Could you check a few things on this model? Use its own coordinates, in mm. Face numbers are marked on the shaded views. A direction names the side the tool comes from. Give positions to 0.01 mm unless a question says otherwise; leave off trailing zeros. Loops run counter-clockwise (first coordinate to the right, second up) from the corner with the lowest first, then second, coordinate; pieces in that order, holes last. Notation, with made-up numbers: (-28, 41) -> (-20, 41) arc R16 ccw to (-20, 46) -> close; hole circle Ø4 at (40, 63). An arc over 180 degrees is marked (long way). Put each result on its own line as item: value.
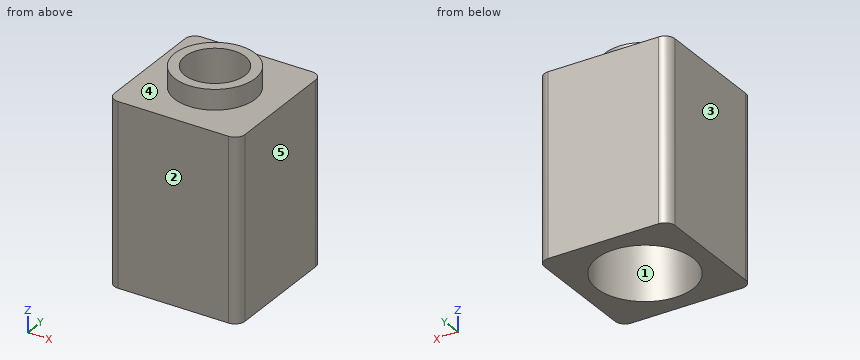
```python
from build123d import *

# Parameters (mm, degrees)
SKETCH2_R           = 1.5
BOSS_EXTRUDE1_DEPTH = 10
SKETCH3_R           = 2
CUT_EXTRUDE1_DEPTH  = 1
SKETCH4_R           = 2.4
CUT_EXTRUDE2_DEPTH  = 8


with BuildPart() as part:
    # Sketch2 → Boss-Extrude1 (new body)
    with BuildSketch(Plane(origin=(0, 0, -57.465471353), x_dir=(-1, 0, 0), z_dir=(0, 0, -1))):
        with BuildLine():
            Line((-6.490457264, -35.078386779), (-0.990457264, -35.078386779))
            ThreePointArc((-0.990457264, -35.078386779), (-0.636903873, -34.931940169), (-0.490457264, -34.578386779))
            Line((-0.490457264, -34.578386779), (-0.490457264, -29.078386779))
            ThreePointArc((-0.490457264, -29.078386779), (-0.636903873, -28.724833388), (-0.990457264, -28.578386779))
            Line((-0.990457264, -28.578386779), (-6.490457264, -28.578386779))
            ThreePointArc((-6.490457264, -28.578386779), (-6.844010654, -28.724833388), (-6.990457264, -29.078386779))
            Line((-6.990457264, -29.078386779), (-6.990457264, -34.578386779))
            ThreePointArc((-6.990457264, -34.578386779), (-6.844010654, -34.931940169), (-6.490457264, -35.078386779))
        make_face()
        with Locations((-3.740457264, -31.828386779)):
            Circle(SKETCH2_R, mode=Mode.SUBTRACT)
    extrude(amount=BOSS_EXTRUDE1_DEPTH)

    # Sketch3 → Cut-Extrude1 (cut)
    with BuildSketch(Plane(origin=(0, 0, -57.465471353), x_dir=(-1, 0, 0), z_dir=(0, 0, -1))):
        with BuildLine():
            Line((-0.990457264, -28.578386779), (-6.490457264, -28.578386779))
            ThreePointArc((-6.490457264, -28.578386779), (-6.844010654, -28.724833388), (-6.990457264, -29.078386779))
            Line((-6.990457264, -29.078386779), (-6.990457264, -34.578386779))
            ThreePointArc((-6.990457264, -34.578386779), (-6.844010654, -34.931940169), (-6.490457264, -35.078386779))
            Line((-6.490457264, -35.078386779), (-0.990457264, -35.078386779))
            ThreePointArc((-0.990457264, -35.078386779), (-0.636903873, -34.931940169), (-0.490457264, -34.578386779))
            Line((-0.490457264, -34.578386779), (-0.490457264, -29.078386779))
            ThreePointArc((-0.490457264, -29.078386779), (-0.636903873, -28.724833388), (-0.990457264, -28.578386779))
        make_face()
        with Locations((-3.740457264, -31.828386779)):
            Circle(SKETCH3_R, mode=Mode.SUBTRACT)
    extrude(amount=CUT_EXTRUDE1_DEPTH, mode=Mode.SUBTRACT)

    # Sketch4 → Cut-Extrude2 (cut)
    with BuildSketch(Plane(origin=(0, 0, -67.465471353), x_dir=(-1, 0, 0), z_dir=(0, 0, -1))):
        with Locations((-3.740457264, -31.828386779)):
            Circle(SKETCH4_R)
    extrude(amount=-CUT_EXTRUDE2_DEPTH, mode=Mode.SUBTRACT)


solid = part.part
```
1. I'm going to push flat-ended pins straight in: pin 1 (1.4 mm diameter, centred on x = 3, y = -31, fed in from -Z); pin 2 (1 mm diameter, centred on x = 4.5, y = -31.5, fed in from +Z). Where does each tip first touch, or does it pass through?
Recorded:
pin 1: stops at z = -59.47
pin 2: passes through
2. For the marked faces 4 and 5, which set-ups out of +Z, -Z, +X, -X, +Y, -Y let a thin tool reach every point of the face, with its end or its side?
Recorded:
face 4: +Z
face 5: +Z, -Z, +X, +Y, -Y
3. If we section it at A-A (x = 4): List the corners of the cut face in (y, z) for me, then the cut area to 3 significant figures.
Recorded:
outline: (-35.08, -67.47) -> (-34.21, -67.47) -> (-34.21, -59.47) -> (-33.31, -59.47) -> (-33.31, -57.47) -> (-33.81, -57.47) -> (-33.81, -58.47) -> (-35.08, -58.47) -> close; (-30.35, -59.47) -> (-29.44, -59.47) -> (-29.44, -67.47) -> (-28.58, -67.47) -> (-28.58, -58.47) -> (-29.85, -58.47) -> (-29.85, -57.47) -> (-30.35, -57.47) -> close
area: 18.4 mm^2
4. If we section it at B-B (y = -31): List the corners of the cut face in (x, z) for me.
Recorded:
outline: (0.49, -67.47) -> (1.49, -67.47) -> (1.49, -59.47) -> (2.49, -59.47) -> (2.49, -57.47) -> (1.92, -57.47) -> (1.92, -58.47) -> (0.49, -58.47) -> close; (4.99, -59.47) -> (5.99, -59.47) -> (5.99, -67.47) -> (6.99, -67.47) -> (6.99, -58.47) -> (5.56, -58.47) -> (5.56, -57.47) -> (4.99, -57.47) -> close
5. I need wall thicknesses on line 1 (X direction, y = -31.75, z = -64); line 2 (Y direction, x = 4, z = -59); line 3 (X direction, y = -30.75, z = -66.25). Which ranges of each line are inside material? Lowest first, please.
Recorded:
line 1: x = 0.49 to 1.34, 6.14 to 6.99
line 2: y = -35.08 to -33.31, -30.35 to -28.58
line 3: x = 0.49 to 1.6, 5.88 to 6.99
6. If we section it at D-D (y = -34): List the corners of the cut face in (x, z) for me, then the cut area to 3 significant figures.
Recorded:
outline: (0.49, -67.47) -> (2.72, -67.47) -> (2.72, -59.47) -> (4.76, -59.47) -> (4.76, -67.47) -> (6.99, -67.47) -> (6.99, -58.47) -> (0.49, -58.47) -> close
area: 42.2 mm^2
7. If we section it at C-C (z = -66.75): List the corners of the cut face in (x, y) for me.
Recorded:
outline: (0.49, -34.58) arc R0.5 ccw to (0.99, -35.08) -> (6.49, -35.08) arc R0.5 ccw to (6.99, -34.58) -> (6.99, -29.08) arc R0.5 ccw to (6.49, -28.58) -> (0.99, -28.58) arc R0.5 ccw to (0.49, -29.08) -> close; hole circle Ø4.8 at (3.74, -31.83)
8. Thinking about a two-plate mould opening in Y: for the marked faces 1, 2 and 3, which applies, pulls with the +Y half, pulls with the -Y half, needs draft (parallel to the pull), parting line crosses it, or undercut?
Recorded:
face 1: undercut
face 2: pulls with the -Y half
face 3: needs draft
